Check sheet for the modelled part. Datum: model origin and axes. Units: mm. A direction names the side the tool comes from. Round coordinates to 2 decimals unless told otherwise and drop trailing zeros. Write each loop counter-clockwise with the first axis right and the second up, starting at its lowest first coordinate (ties: lowest second). Pieces come first, ordered by that corner, then holes. Notation, with made-up numbers: (9, 72.25) -> (20, 72.25) arc R30 ccw to (20, 97.25) -> close; hole circle Ø1 at (5, -25). An arc over 180 degrees is marked (long way). Write item = value, one per line.
from build123d import *

# Parameters (mm, degrees)
F0_R     = 14
F1_DEPTH = 140
F3_DEPTH = 25
F5_DEPTH = 25


with BuildPart() as f1:
    # F0 (on Front) → F1 (new body)
    with BuildSketch(Plane.XZ):
        Circle(F0_R)
    extrude(amount=F1_DEPTH)

    # F2 (on Front) → F3 (join)
    with BuildSketch(Plane.XZ):
        Polygon((2, 10), (-2, 10), (-2, 2), (-10, 2), (-10, -2), (-2, -2), (-2, -10), (2, -10), (2, -2), (10, -2), (10, 2), (2, 2), align=None)
    extrude(amount=-F3_DEPTH)

    # F4 (on face) → F5 (join)
    with BuildSketch(Plane.XZ.offset(140)):
        Polygon((-2, 2), (-10, 2), (-10, -2), (-2, -2), (-2, -10), (2, -10), (2, -2), (10, -2), (10, 2), (2, 2), (2, 10), (-2, 10), align=None)
    extrude(amount=F5_DEPTH)


solid = f1.part
(1) Access from +Z, -Z, +X, -X, +Y, -Y to the whole of each face (thin tool, end or side, straight path). Record for faces 1 (the flat face through (2, 12, 6)), 2 (the flat face through (-2, 12, 6)), 3 (the flat face through (-2, -152, -6)).
Worked answers:
face_1 = +Z, +X, +Y
face_2 = +Z, -X, +Y
face_3 = -Z, -X, -Y
(2) Material ranges on L1, parallel to Y at x = -11.5, z = -6.75; L2, parallel to Z at x = -1, y = -34; L3, parallel to X at y = -18, z = 9, recorded low to high. Write a range as [from, to].
Worked answers:
L1 = [-140, 0]
L2 = [-13.96, 13.96]
L3 = [-10.72, 10.72]
(3) Sectioned sample at C-C on y = -70. Enter the section's corners in (x, z), then the cut area to 3 significant figures.
Worked answers:
outline = circle Ø28 at (0, 0)
area = 616 mm²
(4) Go/stop test with flat-tipped pins: P1, Ø6.5, axis at x = 5.5, y = 6.5, coming from the -Z side; P2, Ø9, axis at x = 5.5, y = -153.5, coming from the +Z side; P3, Ø9, axis at y = -152.5, z = 6, coming from the +X side. Record where each tip stops, or that it passes through.
Worked answers:
P1 = -2
P2 = 10
P3 = 10
(5) Sectioned sample at A-A on x = 0. Enter the section's corners in (y, z), then the cut area to 3 significant figures.
Worked answers:
outline = (-165, -10) -> (-140, -10) -> (-140, -14) -> (0, -14) -> (0, -10) -> (25, -10) -> (25, 10) -> (0, 10) -> (0, 14) -> (-140, 14) -> (-140, 10) -> (-165, 10) -> close
area = 4,920 mm²
(6) Sectioned sample at B-B on z = 0. Enter the section's corners in (x, y), then the cut area to 3 significant figures.
Worked answers:
outline = (-14, -140) -> (-10, -140) -> (-10, -165) -> (10, -165) -> (10, -140) -> (14, -140) -> (14, 0) -> (10, 0) -> (10, 25) -> (-10, 25) -> (-10, 0) -> (-14, 0) -> close
area = 4,920 mm²
